Geometry check sheet. Reference: the model listing, model coordinates, mm. Face numbers are marked on the shaded views. A direction names the side the tool comes from. Round coordinates to 2 decimals unless told otherwise and drop trailing zeros. Order: outer loops, then holes, each group sorted by start corner. A loop starts at its lowest first (then second) coordinate and runs counter-clockwise, first axis right, second up. Notation, with made-up numbers: (-24.75, 60) -> (27.25, 60) arc R26 ccw to (27.25, 89) -> close; hole circle Ø1 at (-10, -0.75). An arc over 180 degrees is marked (long way). Use a Markdown table: item, result. Add a question column.
Item 1: Set-up check for the marked faces 1, 2 and 3: record each of +Z, -Z, +X, -X, +Y, -Y from which the full face is reachable in a straight line by a thin tool's end or side.
Item 2: Material ranges on probe 1 along X at (y, z) = (4.7, 18.85) (3 decimals); probe 2 along Y at (x, z) = (-1.5, 18); probe 3 along Z at (x, y) = (7.55, 4.05) (3 decimals), recorded low to high. Write a range as [from, to].
Item 3: Gauge pin test, flat ends, axial feed: pin 1 Ø2 at (x, z) = (8, 16.5) entering from -Y; pin 2 Ø2 at (x, z) = (7.55, 18.85) entering from +Y; pin 3 Ø0.5 at (x, z) = (17, 9.5) entering from -Y; pin 4 Ø1.5 at (x, y) = (12, 2) entering from +Z. Record the tip position at first contact, or that the pin passes through.
Item 4: Sectioned sample at C-C, the plane y = 4.05. Record the cut outline in (x, z) (3 decimals).
Item 5: Mould release check, pull along X, two halves, no side actions. Record for the marked faces 4, 5, 6 and 7: pulls with the +X half, pulls with the -X half, needs draft (parallel to the pull), parting line crosses it, or undercut.
Item 6: Sectioned sample at B-B, the plane z = 18.85. Record the cut outline in (x, y) (3 decimals), and give its area (3 significant figures).
from build123d import *

# Parameters (mm, degrees)
CYLINDER001_R          = 1
CYLINDER001_DEPTH      = 10
CYLINDER001_ROLL_ANGLE = 90
ARRAY_X_COUNT          = 2
ARRAY_X_PITCH          = 19.6
BOX_W                  = 19.6
BOX_H                  = 5
BOX_DEPTH              = 10.7
CYLINDER_R             = 1.825
CYLINDER_DEPTH         = 10
CYLINDER_ROLL_ANGLE    = 90
BOX001_W               = 19.6
BOX001_H               = 1.6
BOX001_DEPTH           = 17.5
CHAMFER_SIZE           = 2
POCKET_DEPTH           = 50


with BuildPart() as array:
    # Cylinder001 → Cylinder001 (new body)
    with BuildSketch(Plane.XY):
        Circle(CYLINDER001_R)
    extrude(amount=CYLINDER001_DEPTH)


with BuildPart() as array_1:
    # Cylinder001 roll: moved
    add(array.part.rotate(Axis((0, 0, 0), (1, 0, 0)), CYLINDER001_ROLL_ANGLE))


with BuildPart() as array_2:
    # Cylinder001 placement: moved
    add(array_1.part.moved(Location((0, 4.3, 5.35))))

    # Array X: Array ×2


with BuildPart() as array_3:
    add(array_2.part)
    with Locations(*[(i * ARRAY_X_PITCH, 0, 0) for i in range(1, ARRAY_X_COUNT)]):
        add(array_2.part)


with BuildPart() as cubo:
    # Box → Box (new body)
    with BuildSketch(Plane.XY):
        with Locations((9.8, 2.5)):
            Rectangle(BOX_W, BOX_H)
    extrude(amount=BOX_DEPTH)


with BuildPart() as cilindro:
    # Cylinder → Cylinder (new body)
    with BuildSketch(Plane.XY):
        Circle(CYLINDER_R)
    extrude(amount=CYLINDER_DEPTH)


with BuildPart() as cilindro_1:
    # Cylinder roll: moved
    add(cilindro.part.rotate(Axis((0, 0, 0), (1, 0, 0)), CYLINDER_ROLL_ANGLE))


with BuildPart() as cilindro_2:
    # Cylinder placement: moved
    add(cilindro_1.part.moved(Location((9.8, 10, 14.85))))


with BuildPart() as obj1:
    # Box001 → Box001 (new body)
    with BuildSketch(Plane(origin=(0, 3.4, 0), x_dir=(1, 0, 0), z_dir=(0, 0, 1))):
        with Locations((9.8, 0.8)):
            Rectangle(BOX001_W, BOX001_H)
    extrude(amount=BOX001_DEPTH)

    # Chamfer
    chamfer_edges = [obj1.edges().sort_by_distance(p)[0] for p in [
        (0, 4.2, 17.5),
        (19.6, 4.2, 17.5),
    ]]
    chamfer(chamfer_edges, length=CHAMFER_SIZE)

    # Cut: cut Cilindro
    add(cilindro_2.part, mode=Mode.SUBTRACT)

    # Fusion: union Cubo
    add(cubo.part)

    # Sketch → Pocket (cut, symmetric)
    with BuildSketch(Plane.YZ.offset(19.6)):
        Polygon((3.400024, 10.700153), (-0.022797, 10.708087), (-0.047538, 10.466272), align=None)
        Polygon((-0.28005, 0.647481), (0.962411, -0.006446), (-0.389037, -0.137231), align=None)
        Polygon((3.403737, -0.006446), (5.125743, 0.21153), (5.191135, -0.377004), align=None)
    extrude(amount=POCKET_DEPTH, both=True, mode=Mode.SUBTRACT)

    # Cut001: cut Array
    add(array_3.part, mode=Mode.SUBTRACT)


with BuildPart() as obj1_1:
    # Cut001 placement: moved
    add(obj1.part.moved(Location((-2.25, 0, 4))))


solid = obj1_1.part
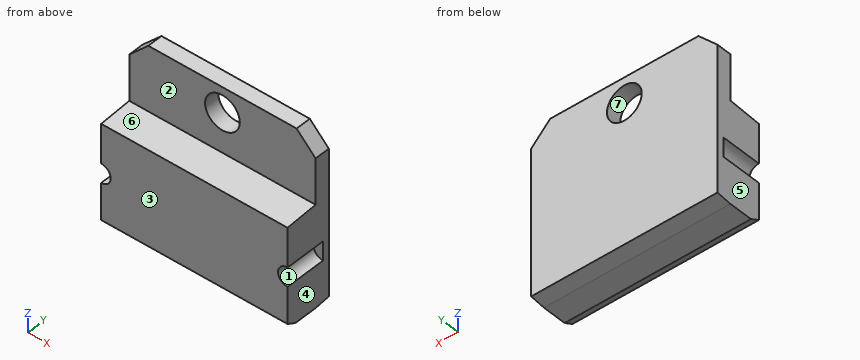
Found:
| question | item | result |
|---|---|---|
| 1 | face 1 | +X, -Y |
| 1 | face 2 | +Z, +X, -X, -Y |
| 1 | face 3 | +Z, -Z, +X, -X, -Y |
| 2 | probe 1 | x = [-2.25, 5.725], [9.375, 17.35] |
| 2 | probe 2 | y = [3.4, 5] |
| 2 | probe 3 | z = [4.075, 17.025], [20.675, 21.5] |
| 3 | pin 1 | stops at y = 3.4 |
| 3 | pin 2 | passes through |
| 3 | pin 3 | stops at y = 4.3 |
| 3 | pin 4 | stops at z = 14.66 |
| 4 | outline | (-2.25, 4.075) -> (17.35, 4.075) -> (17.35, 8.35) arc R1 cw to (17.35, 10.35) -> (17.35, 19.5) -> (15.35, 21.5) -> (-0.25, 21.5) -> (-2.25, 19.5) -> (-2.25, 10.35) arc R1 cw to (-2.25, 8.35) -> close; hole circle Ø3.65 at (7.55, 18.85) |
| 5 | face 4 | pulls with the +X half |
| 5 | face 5 | pulls with the -X half |
| 5 | face 6 | needs draft |
| 5 | face 7 | undercut |
| 6 | outline | (-2.25, 3.4) -> (5.725, 3.4) -> (5.725, 5) -> (-2.25, 5) -> close; (9.375, 3.4) -> (17.35, 3.4) -> (17.35, 5) -> (9.375, 5) -> close |
| 6 | area | 25.5 mm2 |
